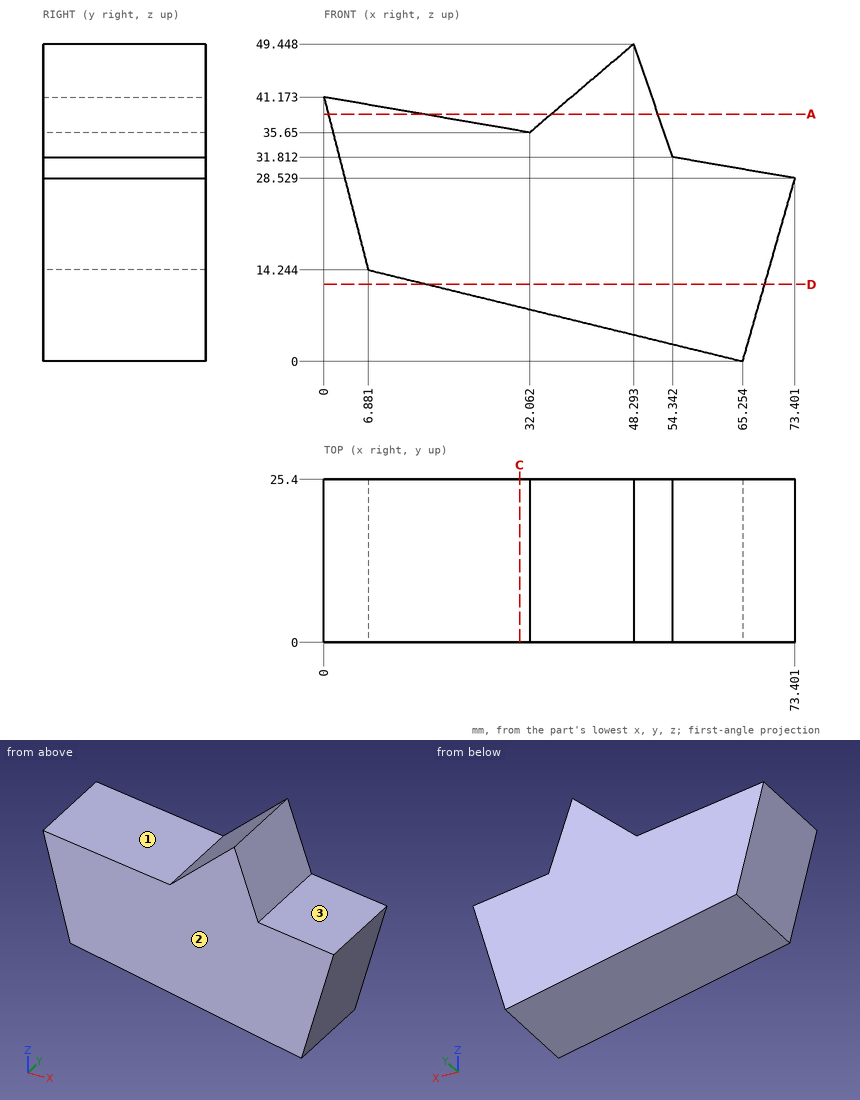
Could you check a few things on this drawing? It's one solid part, dimensions in mm from its lowest x, y, z. Round coordinates to 2 decimals unless told otherwise and drop trailing zeros. Write each loop counter-clockwise with the first axis right and the second up, starting at its lowest first coordinate (ties: lowest second). Pieces come first, ordered by that corner, then holes. Notation, with made-up numbers: M 69.5,82.5 L 96.5,82.5 A28 cw 96.5,103.5 Z; hole C 42.25,65.25 d3. An arc over 180 degrees is marked long. Answer as CSV lines item,"result". Start each with the question number.
1. Suppose I cut it at A-A on z = 38.5. Write out the boundary of the cut face in (x, y), then the cut area to 3 significant figures.
2. Suppose I cut it at D-D on z = 12. Write out the boundary of the cut face in (x, y).
3. I'm going to push flat-ended pins straight in: pin 1 Ø10 at (y, z) = (21.5, 14.5) entering from -X; pin 2 Ø1 at (x, y) = (41, 16) entering from -Z; pin 3 Ø1 at (x, y) = (13.5, 21) entering from -Z. Where does each tip first touch, or does it pass through?
4. Thinking about a two-plate mould opening in X: for the marked faces 1, 2 and 3, which applies, released by +X, released by -X, zero draft, split by the parting line, or undercut?
5. I need wall thicknesses on probe 1 along X at (y, z) = (5, 35.5); probe 2 along X at (y, z) = (15, 35); probe 3 along Z at (x, y) = (58.5, 23) (1 decimal). Which ranges of each line are inside material? Lowest first, please.
6. Suppose I cut it at C-C on x = 30.5. Write out the boundary of the cut face in (y, z).
Check result:
1,outline,"M 0.68,0 L 15.52,0 L 15.52,25.4 L 0.68,25.4 Z; M 35.41,0 L 52.05,0 L 52.05,25.4 L 35.41,25.4 Z"
1,area,"799 mm2"
2,outline,"M 16.08,0 L 68.68,0 L 68.68,25.4 L 16.08,25.4 Z"
3,pin 1,"stops at x = 5.54"
3,pin 2,"stops at z = 5.8"
3,pin 3,"stops at z = 12.51"
4,face 1,"undercut"
4,face 2,"zero draft"
4,face 3,"released by +X"
5,probe 1,"x = 1.45 to 53.08"
5,probe 2,"x = 1.58 to 53.25"
5,probe 3,"z = 1.6 to 31.1"
6,outline,"M 0,8.48 L 25.4,8.48 L 25.4,35.92 L 0,35.92 Z"
